Read the model definition and answer for the solid it produces. Units are mm, in the model's axes. Face numbers are marked on the shaded views. A direction names the side the tool comes from. Coordinates: 2 decimals unless noted, no trailing zeros. Loops run counter-clockwise (first coordinate to the right, second up) from the corner with the lowest first, then second, coordinate; pieces in that order, holes last. Notation, with made-up numbers: (-23.75, 64.5) -> (20.25, 64.5) arc R12 ccw to (20.25, 69.5) -> close; hole circle Ø10 at (-33.5, 88.25). An arc over 180 degrees is marked (long way). Answer in a Markdown table with one row per item.
```python
from build123d import *

# Parameters (mm, degrees)
F0_W     = 38.1
F0_H     = 38.1
F1_DEPTH = 38.1
F5_DEPTH = 38.1
F7_DEPTH = 38.1
F9_DEPTH = 38.1


with BuildPart() as f1:
    # F0 (on Front) → F1 (new body)
    with BuildSketch(Plane.XZ):
        with Locations((47.4635573444, 19.05)):
            Rectangle(F0_W, F0_H)
    extrude(amount=F1_DEPTH)

    # F4 (on face) → F5 (cut)
    with BuildSketch(Plane.YZ.offset(66.5135573444)):
        Polygon((-31.75, 0), (-38.1, 38.1), (-38.1, 0), align=None)
        Polygon((-6.35, 38.1), (-31.75, 38.1), (-26.67, 19.0584023679), (-21.59, 28.575), (-16.51, 28.575), (-11.43, 19.0584023679), align=None)
        Polygon((0, 0), (0, 38.1), (-6.35, 0), align=None)
        Polygon((-19.05, 15.875), (-25.4, 0), (-12.7, 0), align=None)
    extrude(amount=-F5_DEPTH, mode=Mode.SUBTRACT)

    # F6 (on offset) → F7 (cut)
    with BuildSketch(Plane.XZ.offset(38.1)):
        Polygon((38.4384175691, 22.0491613483), (34.7635573444, 0), (60.1635573444, 0), (55.1432829689, 22.0491613483), (50.4643332552, 12.2184510259), (44.1477571021, 12.2184510259), align=None)
        Polygon((34.7635573444, 38.1), (28.4135573444, 38.1), (28.4135573444, 0), align=None)
        Polygon((54.1253941298, 38.1), (41.1135573444, 38.1), (47.4635573444, 27.2768866271), align=None)
        Polygon((60.4753941298, 38.1), (66.5135573444, 0), (66.5135573444, 38.1), align=None)
    extrude(amount=-F7_DEPTH, mode=Mode.SUBTRACT)

    # F8 (on offset) → F9 (cut)
    with BuildSketch(Plane.XY.offset(38.1)):
        Polygon((59.8412752151, 0), (52.2212752151, 0), (52.2212752151, -12.7), (52.2212752151, -25.3993560767), (59.8412752151, -25.3993560767), (59.8412752151, -12.6993560767), align=None)
    extrude(amount=-F9_DEPTH, mode=Mode.SUBTRACT)


solid = f1.part
```
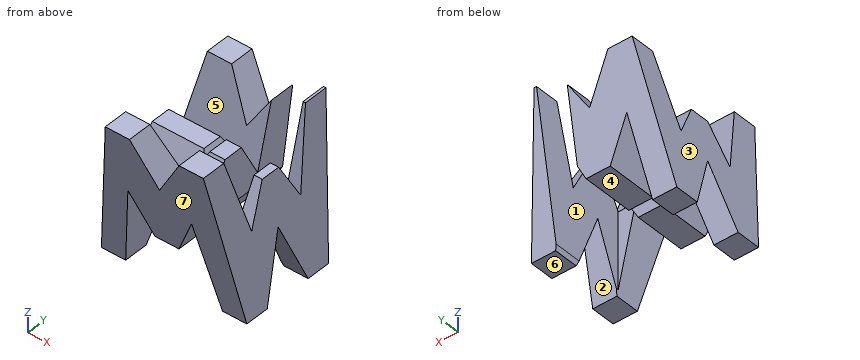
1. A tool of negligible diameter and unlimited length cuts with its end or side. For the marked faces 1, 2, 3 and 4, from which of +Z, -Z, +X, -X, +Y, -Y can it reach the whole face along a straight path? Write none if from no direction.
A:
| item | result |
|---|---|
| face 1 | +Z, -Z, +Y |
| face 2 | -Z, +X, -X |
| face 3 | +Z, -X, +Y, -Y |
| face 4 | -Z, +Y, -Y |
2. A cutting plane is placed at A-A on z = 13.5. Give the vertices of the cut face in (x, y), and give its area (3 significant figures).
A:
| item | result |
|---|---|
| outline | (30.66, -34) -> (37.01, -34) -> (37.01, -20) -> (30.66, -20) -> close; (30.66, -18.1) -> (37.01, -18.1) -> (37.01, -4.1) -> (30.66, -4.1) -> close; (43.4, -34) -> (51.07, -34) -> (51.07, -20) -> (43.4, -20) -> close; (43.4, -18.1) -> (51.07, -18.1) -> (51.07, -4.1) -> (43.4, -4.1) -> close; (57.09, -34) -> (64.37, -34) -> (64.37, -20) -> (59.84, -20) -> (59.84, -25.4) -> (57.09, -25.4) -> close; (59.84, -18.1) -> (64.37, -18.1) -> (64.37, -4.1) -> (59.84, -4.1) -> close |
| area | 543 mm2 |
3. A cutting plane is placed at C-C on z = 30.5. Give the vertices of the cut face in (x, y), and give its area (3 significant figures).
A:
| item | result |
|---|---|
| outline | (33.5, -36.83) -> (45.57, -36.83) -> (45.57, -29.72) -> (33.5, -29.72) -> close; (33.5, -8.38) -> (45.57, -8.38) -> (45.57, -1.27) -> (33.5, -1.27) -> close; (49.45, -36.83) -> (61.68, -36.83) -> (61.68, -29.72) -> (49.45, -29.72) -> close; (49.45, -8.38) -> (52.22, -8.38) -> (52.22, -1.27) -> (49.45, -1.27) -> close; (59.84, -8.38) -> (61.68, -8.38) -> (61.68, -1.27) -> (59.84, -1.27) -> close |
| area | 292 mm2 |
4. A cutting plane is placed at D-D on y = -34.5. Give the vertices of the cut face in (x, z), and give its area (3 significant figures).
A:
| item | result |
|---|---|
| outline | (31.16, 16.5) -> (37.51, 16.5) -> (38.44, 22.05) -> (41.66, 16.5) -> (52.5, 16.5) -> (55.14, 22.05) -> (56.41, 16.5) -> (63.9, 16.5) -> (60.48, 38.1) -> (54.13, 38.1) -> (47.46, 27.28) -> (41.11, 38.1) -> (34.76, 38.1) -> close |
| area | 538 mm2 |
5. Find the intervals of material crossed by probe 1 along X at (y, z) = (-30, 13); probe 2 along X at (y, z) = (-20, 15); probe 3 along Y at (x, z) = (60.5, 22.5), in increasing order.
A:
| item | result |
|---|---|
| probe 1 | x = 30.58 to 36.93, 43.69 to 50.84, 57.2 to 64.45 |
| probe 2 | x = 30.91 to 37.26, 42.53 to 51.79, 59.84 to 64.14 |
| probe 3 | y = -35.5 to -27.59, -24.83 to -13.27, -10.51 to -2.6 |
6. The mould has two halves that part along Y. Classify the marked faces 5, 6 and 7: pulls with the +Y half, pulls with the -Y half, needs draft (parallel to the pull), parting line crosses it, or undercut.
A:
| item | result |
|---|---|
| face 5 | undercut |
| face 6 | needs draft |
| face 7 | pulls with the -Y half |
7. A cutting plane is placed at B-B on y = -8.5. Give the vertices of the cut face in (x, z), and give its area (3 significant figures).
A:
| item | result |
|---|---|
| outline | (28.41, 0) -> (34.76, 0) -> (38.44, 22.05) -> (44.15, 12.22) -> (50.46, 12.22) -> (52.22, 15.91) -> (52.22, 30.04) -> (49.16, 30.04) -> (47.46, 27.28) -> (45.84, 30.04) -> (33.42, 30.04) -> close; (59.84, 1.42) -> (60.16, 0) -> (66.51, 0) -> (61.75, 30.04) -> (59.84, 30.04) -> close |
| area | 524 mm2 |
8. Given pin 1 Ø1 at (y, z) = (-4.5, 26) entering from +X; pin 2 Ø3 at (x, y) = (46, -13) entering from -Z; pin 3 Ø1.1 at (x, y) = (61.5, -20) entering from +Z (3 decimals), each flat-ended and moving along its own axis, determine where each tip first touches the part or whether it passes through.
A:
| item | result |
|---|---|
| pin 1 | stops at x = 62.47 |
| pin 2 | stops at z = 12.22 |
| pin 3 | stops at z = 28.575 |
